```python
from build123d import *

# Parameters (mm, degrees)
SKETCH2_W           = 48
SKETCH2_H           = 45
BOSS_EXTRUDE1_DEPTH = 8
BOSS_EXTRUDE2_DEPTH = 8
CUT_EXTRUDE1_START  = -8
SKETCH4_R           = 18
CUT_EXTRUDE1_DEPTH  = 3
SKETCH5_R           = 4
SKETCH5_R_2         = 1
CUT_EXTRUDE2_DEPTH  = 46
SKETCH6_W           = 25
SKETCH6_H           = 45
BOSS_EXTRUDE3_DEPTH = 60
FILLET7_R           = 5
SKETCH7_W           = 12
SKETCH7_H           = 45
BOSS_EXTRUDE4_DEPTH = 45
FILLET10_R          = 22
SKETCH8_R           = 18
CUT_EXTRUDE3_DEPTH  = 3
SKETCH9_R           = 4
SKETCH9_R_2         = 1
CUT_EXTRUDE4_DEPTH  = 28
CUT_EXTRUDE5_DEPTH  = 46
FILLET11_R          = 5
FILLET12_R          = 7


with BuildPart() as part:
    # Sketch2 → Boss-Extrude1 (new body)
    with BuildSketch(Plane(origin=(0, 0, 0), x_dir=(1, 0, 0), z_dir=(0, 1, 0))):
        Rectangle(SKETCH2_W, SKETCH2_H)
    extrude(amount=BOSS_EXTRUDE1_DEPTH)

    # Sketch3 → Boss-Extrude2 (add)
    with BuildSketch(Plane(origin=(24, 0, 0), x_dir=(0, 0, -1), z_dir=(1, 0, 0))):
        with BuildLine():
            Line((-22.5, 0), (22.5, 0))
            Line((22.5, 0), (22.5, -23))
            ThreePointArc((22.5, -23), (16.056349186, -38.556349186), (0.5, -45))
            Line((0.5, -45), (-0.5, -45))
            ThreePointArc((-0.5, -45), (-16.056349186, -38.556349186), (-22.5, -23))
            Line((-22.5, -23), (-22.5, 0))
        make_face()
    extrude(amount=-BOSS_EXTRUDE2_DEPTH)

    # Sketch4 → Cut-Extrude1 (cut)
    with BuildSketch(Plane.ZY.offset(-16).offset(CUT_EXTRUDE1_START)):
        with Locations((0, -22.5)):
            Circle(SKETCH4_R)
    extrude(amount=CUT_EXTRUDE1_DEPTH, mode=Mode.SUBTRACT)

    # Sketch5 → Cut-Extrude2 (cut, through all)
    with BuildSketch(Plane(origin=(21, 0, 0), x_dir=(0, 0, -1), z_dir=(1, 0, 0))):
        with Locations((0, -22.5)):
            Circle(SKETCH5_R)
        with Locations((0, -11.5)):
            Circle(SKETCH5_R_2)
        with Locations((11, -22.5)):
            Circle(SKETCH5_R_2)
        with Locations((0, -33.5)):
            Circle(SKETCH5_R_2)
        with Locations((-11, -22.5)):
            Circle(SKETCH5_R_2)
    extrude(amount=-CUT_EXTRUDE2_DEPTH, mode=Mode.SUBTRACT)

    # Mirror1: part across plane


with BuildPart() as part_1:
    add(part.part)
    add(part.part.mirror(Plane(origin=(0, 0, 0), x_dir=(0, 0, 1), z_dir=(1, 0, 0))))

    # Sketch6 → Boss-Extrude3 (add)
    with BuildSketch(Plane(origin=(0, 8, 0), x_dir=(1, 0, 0), z_dir=(0, 1, 0))):
        Rectangle(SKETCH6_W, SKETCH6_H)
    extrude(amount=BOSS_EXTRUDE3_DEPTH)

    # Fillet7
    fillet7_edges = [part_1.edges().sort_by_distance(p)[0] for p in [
        (16, 0, 0),
        (-16, 0, 0),
    ]]
    fillet(fillet7_edges, radius=FILLET7_R)

    # Sketch7 → Boss-Extrude4 (add)
    with BuildSketch(Plane(origin=(0, 68, 0), x_dir=(1, 0, 0), z_dir=(0, 1, 0))):
        Rectangle(SKETCH7_W, SKETCH7_H)
    extrude(amount=BOSS_EXTRUDE4_DEPTH)

    # Fillet10
    fillet10_edges = [part_1.edges().sort_by_distance(p)[0] for p in [
        (0, 113, -22.5),
        (0, 113, 22.5),
    ]]
    fillet(fillet10_edges, radius=FILLET10_R)

    # Sketch8 → Cut-Extrude3 (cut)
    with BuildSketch(Plane.ZY.offset(6)):
        with Locations((0.5, 90.5)):
            Circle(SKETCH8_R)
    extrude(amount=-CUT_EXTRUDE3_DEPTH, mode=Mode.SUBTRACT)

    # Sketch9 → Cut-Extrude4 (cut, through all)
    with BuildSketch(Plane.ZY.offset(3)):
        with Locations((0.5, 90.5)):
            Circle(SKETCH9_R)
        with Locations((0.5, 101.5)):
            Circle(SKETCH9_R_2)
        with Locations((11.5, 90.5)):
            Circle(SKETCH9_R_2)
        with Locations((0.5, 79.5)):
            Circle(SKETCH9_R_2)
        with Locations((-10.5, 90.5)):
            Circle(SKETCH9_R_2)
    extrude(amount=-CUT_EXTRUDE4_DEPTH, mode=Mode.SUBTRACT)

    # Sketch10 → Cut-Extrude5 (cut, through all)
    with BuildSketch(Plane(origin=(0, 0, -22.5), x_dir=(-1, 0, 0), z_dir=(0, 0, -1))):
        with BuildLine():
            Line((12.5, 68), (6, 68))
            add(Edge.make_bspline(
                [(6, 68), (4.938641011, 55.683018677), (12.5, 45.493141657)],
                knots=[0, 0, 0, 1, 1, 1], degree=2))
            Line((12.5, 45.493141657), (12.5, 68))
        make_face()
        with BuildLine():
            Line((-6, 68), (-12.5, 68))
            Line((-12.5, 68), (-12.5, 45.493141657))
            add(Edge.make_bspline(
                [(-6, 68), (-4.938641011, 55.683018677), (-12.5, 45.493141657)],
                knots=[0, 0, 0, 1, 1, 1], degree=2))
        make_face()
    extrude(amount=-CUT_EXTRUDE5_DEPTH, mode=Mode.SUBTRACT)

    # Fillet11
    fillet11_edges = [part_1.edges().sort_by_distance(p)[0] for p in [
        (24, 8, 0),
        (-24, 8, 0),
    ]]
    fillet(fillet11_edges, radius=FILLET11_R)

    # Fillet12
    fillet12_edges = [part_1.edges().sort_by_distance(p)[0] for p in [
        (-12.5, 8, 0),
        (12.5, 8, 0),
    ]]
    fillet(fillet12_edges, radius=FILLET12_R)


solid = part_1.part
```
Geometry check sheet. Reference: the model listing, model coordinates, mm. A direction names the side the tool comes from. Coordinates: 2 decimals unless noted, no trailing zeros. Loops run counter-clockwise (first coordinate to the right, second up) from the corner with the lowest first, then second, coordinate; pieces in that order, holes last. Notation, with made-up numbers: (-3.5, -14) -> (10.5, -14) arc R14 cw to (10.5, 1) -> close; hole circle Ø1 at (1.5, -22.75). An arc over 180 degrees is marked (long way). Put each result on its own line as item: value.
1) Tool access check on faces 5 (the flat face through (-16, -25, 5)), 6 (the flat face through (6, 85, 0)), 7 (the cylindrical face through (-4.521, 108.347, -1.843)), 8 (the flat face through (-6, 75, -10)). Record the directions out of +Z, -Z, +X, -X, +Y, -Y that give a thin tool (end or side, any length) a straight path to the whole face; none if there is none.
Result set:
face 5: +Z, -Z, -Y
face 6: +Z, -Z, +X, +Y
face 7: -X
face 8: +Z, -Z, -X, +Y
2) Thickness scan on line 1 (X direction, y = -27, z = -20); line 2 (Z direction, x = -22, y = -22); line 3 (X direction, y = -34, z = -6). Record the ranges inside material, lowest first.
Result set:
line 1: x = -24 to -16, 16 to 24
line 2: z = -22.5 to -17.99, 17.99 to 22.5
line 3: x = -21 to -16, 16 to 21
3) Release check for a two-part mould opening along Z. For faces 1 (the cylindrical face through (18.535, -18.534, 0.521)), 2 (the cylindrical face through (-23, 6, 0)), 3 (the flat face through (0, 33, 22.5)), 4 (the flat face through (21, -22.2, -4.3)) record: released by +Z, released by -Z, zero draft, split by the parting line, or undercut.
Result set:
face 1: undercut
face 2: zero draft
face 3: released by +Z
face 4: undercut
4) Cross-section at B-B on y = 25. Record the boundary of the cut face in (x, z).
Result set:
outline: (-12.5, -22.5) -> (12.5, -22.5) -> (12.5, 22.5) -> (-12.5, 22.5) -> close
5) Gauge pin test, flat ends, axial feed: pin 1 Ø22.5 at (y, z) = (89.5, -7) entering from -X; pin 2 Ø12 at (x, y) = (-17, 82) entering from +Z; pin 3 Ø24.5 at (y, z) = (29, 5) entering from +X; pin 4 Ø1 at (y, z) = (-15, -3.5) entering from -X. Record the tip position at first contact, or that the pin passes through.
Result set:
pin 1: stops at x = -6
pin 2: passes through
pin 3: stops at x = 12.5
pin 4: stops at x = -21
6) Cross-section at A-A on y = 76. Record the boundary of the cut face in (x, z), plus the area to 3 significant figures.
Result set:
outline: (-6, -22.5) -> (6, -22.5) -> (6, 22.5) -> (-6, 22.5) -> (-6, 11.17) -> (-3, 11.17) -> (-3, -10.17) -> (-6, -10.17) -> close
area: 476 mm^2
